from build123d import *

# Parameters (mm, degrees)
BOSS_EXTRUDE1_DEPTH    = 1
F_10_CLEARANCE_HOLE1_D = 5.1054


with BuildPart() as part:
    # Sketch1 → Boss-Extrude1 (new body)
    # profile 1 of 3: a face of its own
    with BuildSketch(Plane(origin=(0, 0, 0), x_dir=(1, 0, 0), z_dir=(0, 1, 0))):
        with BuildLine():
            Line((0.660254038, 5), (-8, 5))
            ThreePointArc((-8, 5), (-13, 0), (-8, -5))
            Line((-8, -5), (2, -5))
            ThreePointArc((2, -5), (-2.829629131, -1.294095226), (-0.5, 4.330127019))
            Line((-0.5, 4.330127019), (0.660254038, 5))
        make_face()
    # profile 2 of 3: a face of its own
    with BuildSketch(Plane(origin=(0, 0, 0), x_dir=(1, 0, 0), z_dir=(0, 1, 0))):
        with BuildLine():
            Line((2, 5), (0.660254038, 5))
            Line((0.660254038, 5), (-0.5, 4.330127019))
            ThreePointArc((-0.5, 4.330127019), (-2.829629131, -1.294095226), (2, -5))
            ThreePointArc((2, -5), (3.294095226, -4.829629131), (4.5, -4.330127019))
            ThreePointArc((4.5, -4.330127019), (6.829629131, 1.294095226), (2, 5))
        make_face()
    # profile 3 of 3: a face of its own
    with BuildSketch(Plane(origin=(0, 0, 0), x_dir=(1, 0, 0), z_dir=(0, 1, 0))):
        with BuildLine():
            Line((10.325317547, 10.580127019), (0.660254038, 5))
            Line((0.660254038, 5), (2, 5))
            ThreePointArc((2, 5), (6.829629131, 1.294095226), (4.5, -4.330127019))
            Line((4.5, -4.330127019), (15.325317547, 1.919872981))
            ThreePointArc((15.325317547, 1.919872981), (17.155444566, 8.75), (10.325317547, 10.580127019))
        make_face()
        with BuildLine():
            ThreePointArc((12.160254038, 2.401923789), (8.062177826, 3.5), (9.160254038, 7.598076211))
            Line((9.160254038, 7.598076211), (11.758330249, 9.098076211))
            ThreePointArc((11.758330249, 9.098076211), (15.856406461, 8), (14.758330249, 3.901923789))
            Line((14.758330249, 3.901923789), (12.160254038, 2.401923789))
        make_face(mode=Mode.SUBTRACT)
    extrude(amount=BOSS_EXTRUDE1_DEPTH)

    # #10 Clearance Hole1 (through all)
    with Locations(Plane(origin=(0, 1, 0), x_dir=(1, 0, 0), z_dir=(0, 1, 0))):
        with Locations((-8, 0)):
            Hole(F_10_CLEARANCE_HOLE1_D / 2)


solid = part.part
Read the model definition and answer for the solid it produces. Units are mm, in the model's axes. A direction names the side the tool comes from. Round coordinates to 2 decimals unless told otherwise and drop trailing zeros. Write each loop counter-clockwise with the first axis right and the second up, starting at its lowest first coordinate (ties: lowest second). Pieces come first, ordered by that corner, then holes. Notation, with made-up numbers: (39, 51.5) - (73, 51.5) arc R17 cw to (73, 81.5) - close; hole circle Ø2 at (40, -39.5). An arc over 180 degrees is marked (long way). One line per question, with ' | ' between items. Start each with the question number.
1. Section C-C (x = -8.5) is taken. Determine the outline of the cut face in (y, z).
2. Section A-A (z = 0) is taken. Determine the outline of the cut face in (x, y).
3. Find the intervals of material crossed by probe 1 along Z at (x, y) = (-8, 0.6); probe 2 along Z at (x, y) = (-4, 0.7); probe 3 along Z at (x, y) = (-9, 0.6), in increasing order. Write a range as [from, to].
4. Section B-B (y = 0.65) is taken. Determine the outline of the cut face in (x, z).
5. Section D-D (x = -5) is taken. Determine the outline of the cut face in (y, z).
6. For a pull along Z with two mould halves and no side action, classify faces 3 (the face through (-13, 0.5, -0.1)), 4 (the face through (-3.6, 0.5, -5)), 5 (the face through (13.477, 0.493, -3.162)), 6 (the face through (9.837, 0.493, 1.249)) as +Z half, -Z half, draft (parallel to the pull), parting line (faces both ways), or undercut.
7. This flat-tipped pin is pushed along its axis until it touches: pin 1 (3 mm diameter, centred on x = 9.5, z = -3, fed in from +Y). Where does it stop, or does it pass through?
8. For faces 1 (the face through (10.441, 0.493, -8.338)), 2 (the face through (5.56, 0.49, -7.83)), determine the directions among +Z, -Z, +X, -X, +Y, -Y from which every point of the face is accessible in a straight line to the end or side of a thin tool.
Filled in:
1) outline: (0, -4.97) - (1, -4.97) - (1, -2.5) - (0, -2.5) - close; (0, 2.5) - (1, 2.5) - (1, 4.97) - (0, 4.97) - close
2) outline: (-13, 0) - (-10.55, 0) - (-10.55, 1) - (-13, 1) - close; (-5.45, 0) - (12, 0) - (12, 1) - (-5.45, 1) - close
3) probe 1: [-5, -2.55], [2.55, 5] | probe 2: [-5, 5] | probe 3: [-4.9, -2.35], [2.35, 4.9]
4) outline: (-8, -5) - (0.66, -5) - (10.33, -10.58) arc R5 ccw to (15.33, -1.92) - (4.5, 4.33) arc R5 ccw to (2, 5) - (-8, 5) arc R5 ccw to start; hole circle Ø5.11 at (-8, 0); hole (9.16, -7.6) - (11.76, -9.1) arc R3 ccw to (14.76, -3.9) - (12.16, -2.4) arc R3 ccw to start
5) outline: (0, -5) - (1, -5) - (1, 5) - (0, 5) - close
6) face 3: parting line | face 4: -Z half | face 5: undercut | face 6: +Z half
7) pin 1: y = 1
8) face 1: +Y, -Y | face 2: -Z, -X, +Y, -Y
